Design review of the part shown in the three views and the two pictorial views. Dimensions are in mm from the part's minimum x, y and z. Round coordinates to 2 decimals unless told otherwise and drop trailing zeros. Write each loop counter-clockwise with the first axis right and the second up, starting at its lowest first coordinate (ties: lowest second). Pieces come first, ordered by that corner, then holes. Notation, with made-up numbers: (-31, -29) - (-17, -29) arc R28 cw to (-17, 3) - close; hole circle Ø1 at (70.25, 3). An arc over 180 degrees is marked (long way). Use one line per item in the form item = value.
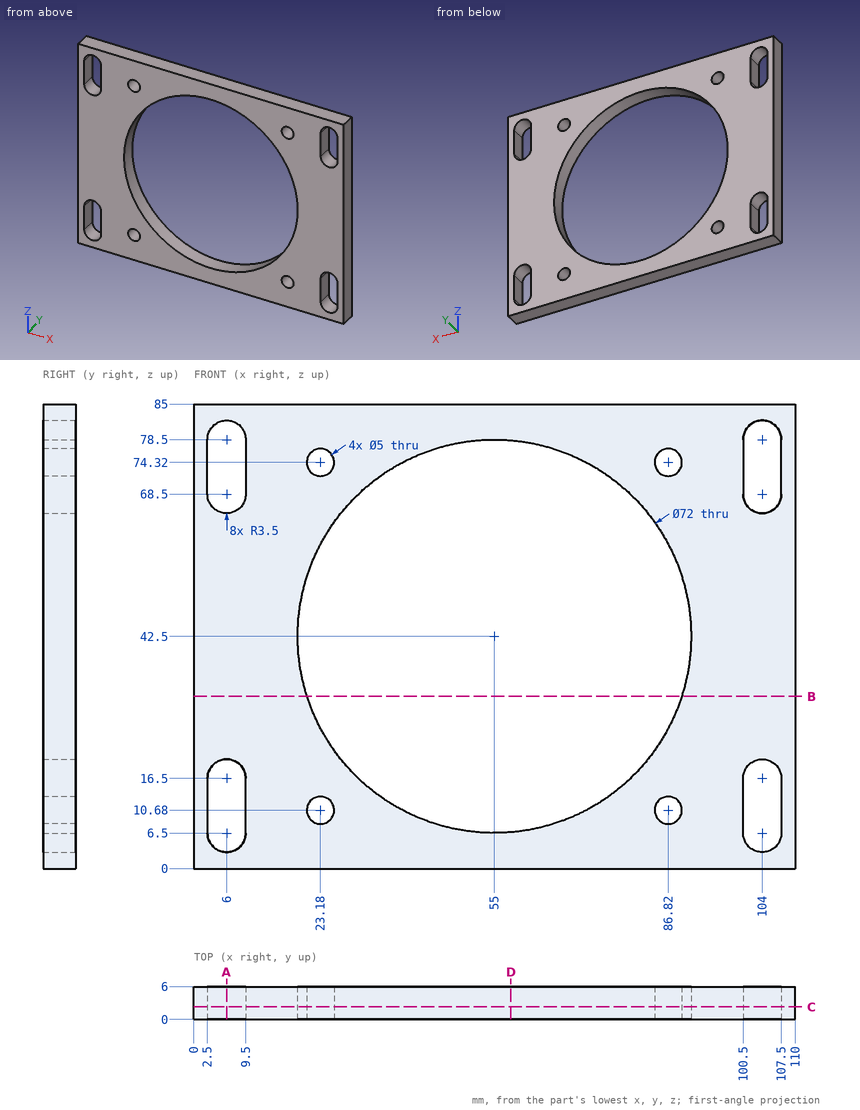
(1) Add section C-C on y = 2.3. Count the separate pieces of the cut face and the enclosed holes in it, then the cut area to 3 significant figures.
Geometry results:
separate_pieces = 1
enclosed_holes = 9
area = 4,770 mm2
(2) Add section D-D on x = 58. Write out the cut boundary in (y, z) (1 decimal).
Geometry results:
outline = (0, 0) - (6, 0) - (6, 6.6) - (0, 6.6) - close; (0, 78.4) - (6, 78.4) - (6, 85) - (0, 85) - close
(3) Add section B-B on z = 31.5. Write out the cut boundary in (x, y).
Geometry results:
outline = (0, 0) - (20.72, 0) - (20.72, 6) - (0, 6) - close; (89.28, 0) - (110, 0) - (110, 6) - (89.28, 6) - close
(4) Add section A-A on x = 6. Write out the cut boundary in (y, z), then the cut area to 3 significant figures.
Geometry results:
outline = (0, 0) - (6, 0) - (6, 3) - (0, 3) - close; (0, 20) - (6, 20) - (6, 65) - (0, 65) - close; (0, 82) - (6, 82) - (6, 85) - (0, 85) - close
area = 306 mm2
(5) To check wall thickness, follow L1, parallel to X at y = 2.25, z = 15; L2, parallel to X at y = 1.65, z = 42.5; L3, parallel to Z at x = 101, y = 4.9. State the ranges of each line that lie inside material, in increasing order.
Geometry results:
L1 = 0 to 2.5, 9.5 to 31.77, 78.23 to 100.5, 107.5 to 110
L2 = 0 to 19, 91 to 110
L3 = 0 to 4.7, 18.3 to 66.7, 80.3 to 85
(6) Insertion check: P1, Ø4, axis at x = 23.18, z = 10.68, coming from the +Y side. The pin has a flat end and moves straight along its axis. Give the tip position at first contact, or say it passes through.
Geometry results:
P1 = through
